Autodesk Inventor part; units mm, degrees
ref_plane "YZ Plane" through (0, 0, 0) normal (1, 0, 0) x (0, 1, 0)
ref_plane "XZ Plane" through (0, 0, 0) normal (0, 1, 0) x (-1, 0, 0)
ref_plane "XY Plane" through (0, 0, 0) normal (0, 0, 1) x (1, 0, 0)
sketch "Náčrt1" plane through (0, 0, 0) normal (0, 0, 1) x (1, 0, 0)
  line L0 (0, 71.1184) -> (0, -73.8108)
  line L1 (-102.6184, 0) -> (105.3108, 0)
  line L2 (-72.5, 50) -> (72.5, 50)
  line L3 (72.5, 50) -> (72.5, -35)
  line L4 (57.5, -50) -> (-72.5, -50)
  line L5 (-72.5, -50) -> (-72.5, 50)
  arc A0 (57.5, -50) -> (72.5, -35) centre (57.5, -35) ccw
  point P0 (0, 0)
  dimension "d2" = 30
  dimension "d37" = 145
  dimension "d38" = 100
extrude "Vysunutí1" add sketch "Náčrt1" along normal blind 21
sketch "Náčrt2" plane through (0, 0, 21) normal (0, 0, 1) x (1, 0, 0)
  line L0 (-72.5, -50) -> (57.5, -50)
  arc A0 (57.5, -50) -> (72.5, -35) centre (57.5, -35) ccw
  line L1 (72.5, -35) -> (72.5, 50)
  line L2 (72.5, 50) -> (-72.5, 50)
  line L3 (-72.5, 50) -> (-72.5, -50)
  circle A1 centre (57.5, -35) radius 15
  line L4 (72.5, -27.3264) -> (72.5, -35)
  line L5 (64.2851, -50) -> (57.5, -50)
  line L6 (72.5, -35) -> (72.5, 50)
  line L7 (72.5, -35) -> (72.5, -35)
  line L8 (72.5, -28.4617) -> (71, -28.4617)
  line L9 (50.9617, -48.5) -> (50.9617, -50)
  point P0 (0, 0)
  point P1 (49.2851, -47.5505)
  point P2 (70.3886, -27.3264)
  point P3 (50.9617, -50)
  dimension "d11" = 1.5
  dimension "d12" = 1.5
extrude "Vysunutí2" cut sketch "Náčrt2" against normal blind 14 contours L9 A1 L0 | A1 A0 | A1 L8 L1
sketch "Náčrt3" plane through (0, 0, 7) normal (0, 0, 1) x (1, 0, 0)
  arc A0 (57.5, -50) -> (72.5, -35) centre (57.5, -35) ccw
  circle A1 centre (57.5, -35) radius 4.25
  line L0 (72.5, -28.4617) -> (72.5, -35)
  line L1 (57.5, -50) -> (50.9617, -50)
  line L2 (71, -28.4617) -> (72.5, -28.4617)
  arc A2 (71, -28.4617) -> (50.9617, -48.5) centre (57.5, -35) ccw
  line L3 (50.9617, -50) -> (50.9617, -48.5)
  point P0 (0, 0)
  dimension "d7" = 8.5
extrude "Vysunutí3" cut sketch "Náčrt3" against normal blind 12 contours A1
fillet "Zaoblení1" radius 2 3 edges at (72.5, 50, 10.5) (-72.5, 50, 10.5) (-72.5, -50, 10.5)
fillet "Zaoblení2" radius 1 2 edges at (71, -28.4617, 14) (50.9617, -48.5, 14)
sketch "Náčrt4" plane through (0, 0, 21) normal (0, 0, 1) x (1, 0, 0)
  arc A0 (50.9617, -49.1129) -> (50.4328, -48.2308) centre (49.9617, -49.1129) ccw
  arc A1 (70.7308, -27.9328) -> (50.4328, -48.2308) centre (57.5, -35) ccw
  arc A2 (70.7308, -27.9328) -> (71.6129, -28.4617) centre (71.6129, -27.4617) ccw
  line L0 (71.6129, -28.4617) -> (72.5, -28.4617)
  line L1 (72.5, -28.4617) -> (72.5, 48)
  arc A3 (72.5, 48) -> (70.5, 50) centre (70.5, 48) ccw
  line L2 (70.5, 50) -> (-70.5, 50)
  arc A4 (-70.5, 50) -> (-72.5, 48) centre (-70.5, 48) ccw
  line L3 (-72.5, 48) -> (-72.5, -48)
  arc A5 (-72.5, -48) -> (-70.5, -50) centre (-70.5, -48) ccw
  line L4 (-70.5, -50) -> (50.9617, -50)
  line L5 (50.9617, -50) -> (50.9617, -49.1129)
  line L6 (-66.5, 44) -> (68.5, 44) construction
  line L7 (68.5, 44) -> (68.5, -44) construction
  line L8 (68.5, -44) -> (-66.5, -44) construction
  line L9 (-66.5, -44) -> (-66.5, 44) construction
  point P0 (0, 0)
  dimension "d14" = 4
  dimension "d15" = 6
  dimension "d16" = 6
  dimension "d17" = 6
sketch "Náčrt5" plane through (0, 0, 21) normal (0, 0, 1) x (1, 0, 0)
  line L0 (-62.1, 26) -> (37.9, 26)
  line L1 (37.9, 26) -> (37.9, -15.5)
  line L2 (37.9, -15.5) -> (-62.1, -15.5)
  line L3 (-62.1, -15.5) -> (-62.1, 26)
  line L4 (-66.5, 44) -> (68.5, 44) construction
  line L5 (-66.5, -44) -> (-66.5, 44) construction
  line L6 (68.5, -44) -> (-66.5, -44) construction
  line L7 (68.5, 44) -> (68.5, -44) construction
  point P0 (0, 0)
  dimension "d18" = 100
  dimension "d19" = 41.5
  dimension "d20" = 18
  dimension "d21" = 4.4
extrude "Vysunutí4" cut sketch "Náčrt5" against normal blind 21
sketch "Náčrt6" plane through (0, 0, 0) normal (0, 0, -1) x (-1, 0, 0)
  line L0 (-37.9, -15.5) -> (-37.9, 26)
  line L1 (-37.9, 26) -> (62.1, 26)
  line L2 (62.1, 26) -> (62.1, -15.5)
  line L3 (62.1, -15.5) -> (-37.9, -15.5)
  arc A0 (70.5, -50) -> (72.5, -48) centre (70.5, -48) ccw
  line L4 (72.5, 48) -> (72.5, -48)
  arc A1 (72.5, 48) -> (70.5, 50) centre (70.5, 48) ccw
  line L5 (-70.5, 50) -> (70.5, 50)
  arc A2 (-70.5, 50) -> (-72.5, 48) centre (-70.5, 48) ccw
  line L6 (-72.5, -35) -> (-72.5, 48)
  arc A3 (-72.5, -35) -> (-57.5, -50) centre (-57.5, -35) ccw
  line L7 (70.5, -50) -> (-57.5, -50)
  circle A4 centre (-57.5, -35) radius 4.25
  arc A5 (-50.4328, -48.2308) -> (-70.7308, -27.9328) centre (-57.5, -35) ccw
  line L8 (0, -73.8108) -> (0, 71.1184)
  line L9 (-105.3108, 0) -> (102.6184, 0)
  line L10 (-68.5, 44) -> (66.5, 44)
  line L11 (66.5, 44) -> (66.5, -44)
  line L12 (66.5, -44) -> (-42.4917, -44)
  line L13 (-68.5, -24.802) -> (-68.5, 44)
  arc A6 (-42.4917, -44) -> (-68.5, -21.3893) centre (-57.5, -35) ccw
  point P0 (0, 0)
  dimension "d24" = 4
  dimension "d25" = 6
  dimension "d26" = 6
  dimension "d27" = 6
  dimension "d28" = 35
extrude "Vysunutí5" cut sketch "Náčrt6" against normal blind 17 contours L3 L8 L12 A6 L13 L9 L0 | L9 L13 L10 L8 L1 L0 | L3 L2 L9 L11 L12 L8 | L8 L10 L11 L9 L2 L1
sketch "Náčrt7" plane through (0, 0, 17) normal (0, 0, -1) x (-1, 0, 0)
  line L0 (-68.5, 44) -> (66.5, 44)
  line L1 (-68.5, -21.3893) -> (-68.5, 44)
  arc A0 (-42.4917, -44) -> (-68.5, -21.3893) centre (-57.5, -35) ccw
  line L2 (66.5, -44) -> (-42.4917, -44)
  line L3 (66.5, 44) -> (66.5, -44)
  line L4 (62.1, -15.5) -> (62.1, 26)
  line L5 (-37.9, -15.5) -> (62.1, -15.5)
  line L6 (-37.9, 26) -> (-37.9, -15.5)
  line L7 (62.1, 26) -> (-37.9, 26)
  line L8 (-40.4, 28.5) -> (64.6, 28.5)
  line L9 (64.6, 28.5) -> (64.6, -18)
  line L10 (64.6, -18) -> (-40.4, -18)
  line L11 (-40.4, -18) -> (-40.4, 28.5)
  point P0 (0, 0)
  dimension "d31" = 2.5
  dimension "d32" = 2.5
  dimension "d33" = 2.5
  dimension "d34" = 2.5
extrude "Vysunutí6" add sketch "Náčrt7" along normal blind 2 contours L8 L9 L10 L11
sketch "Náčrt8" plane through (0, 0, 0) normal (0, 0, -1) x (-1, 0, 0)
  line L0 (-68.5, -21.3893) -> (-68.5, 44)
  line L1 (-68.5, 44) -> (66.5, 44)
  line L2 (66.5, 44) -> (66.5, -44)
  line L3 (66.5, -44) -> (-42.4917, -44)
  arc A0 (-42.4917, -44) -> (-68.5, -21.3893) centre (-57.5, -35) ccw
  arc A1 (70.5, -50) -> (72.5, -48) centre (70.5, -48) ccw
  line L4 (72.5, 48) -> (72.5, -48)
  arc A2 (72.5, 48) -> (70.5, 50) centre (70.5, 48) ccw
  line L5 (-70.5, 50) -> (70.5, 50)
  arc A3 (-70.5, 50) -> (-72.5, 48) centre (-70.5, 48) ccw
  line L6 (-72.5, -35) -> (-72.5, 48)
  arc A4 (-72.5, -35) -> (-57.5, -50) centre (-57.5, -35) ccw
  line L7 (70.5, -50) -> (-57.5, -50)
  circle A5 centre (-57.5, -35) radius 4.25
  point P0 (0, 0)
sketch "Náčrt9" plane through (0, 0, 17) normal (0, 0, -1) x (-1, 0, 0)
  line L0 (-40.4, -18) -> (-40.4, 28.5)
  line L1 (-40.4, 28.5) -> (64.6, 28.5)
  line L2 (64.6, 28.5) -> (64.6, -18)
  line L3 (64.6, -18) -> (-40.4, -18)
  line L4 (-68.5, 44) -> (66.5, 44)
  line L5 (-68.5, -21.3893) -> (-68.5, 44)
  arc A0 (-42.4917, -44) -> (-68.5, -21.3893) centre (-57.5, -35) ccw
  line L6 (66.5, -44) -> (-42.4917, -44)
  line L7 (66.5, 44) -> (66.5, -44)
  line L8 (66.5, -44) -> (-42.4917, -44)
  line L9 (66.5, -44) -> (62, -44)
  line L10 (62, -44) -> (62, -40.5)
  line L11 (62, -40.5) -> (66.5, -40.5)
  line L12 (66.5, -40.5) -> (66.5, -44)
  line L13 (-68.5, 44) -> (-63, 44)
  line L14 (-63, 44) -> (-63, 38.5)
  line L15 (-63, 38.5) -> (-68.5, 38.5)
  line L16 (-68.5, 38.5) -> (-68.5, 44)
  point P0 (0, 0)
  dimension "d48" = 4.5
  dimension "d49" = 3.5
  dimension "d50" = 5.5
  dimension "d51" = 5.5
extrude "Vysunutí7" add sketch "Náčrt9" along normal up to surface (17 mm away) contours L4 L14 L15 L5 | L7 L6 L10 L11
sketch "Náčrt10" plane through (0, 0, 0) normal (0, 0, -1) x (-1, 0, 0)
  circle A0 centre (67, -44.5) radius 3
  circle A1 centre (-68, 45.5) radius 3
  line L0 (-72.5, -35) -> (-72.5, 48)
  line L1 (-70.5, 50) -> (70.5, 50)
  line L2 (70.5, -50) -> (-57.5, -50)
  line L3 (72.5, 48) -> (72.5, -48)
  point P0 (0, 0)
  dimension "d54" = 6
  dimension "d55" = 6
  dimension "d56" = 4.5
  dimension "d57" = 4.5
  dimension "d58" = 5.5
  dimension "d59" = 5.5
sketch "Náčrt11" plane through (0, 0, 21) normal (0, 0, 1) x (1, 0, 0)
  point P0 (0, 0)
  point P1 (-67, -44.5)
  point P2 (68, 45.5)
  point P3 (68, 45.5)
  point P4 (-67, -44.5)
hole "Díra1" at (68, 45.5, 21) at (-67, -44.5, 21) direction (0, 0, -1) diameter 6 depth 17
sketch "Náčrt12" plane through (68, 45.5, 4) normal (0, 0, 1) x (1, 0, 0)
  line L0 (4.5, -73.9617) -> (4.5, 2.5)
  line L1 (2.5, 4.5) -> (-138.5, 4.5)
  circle A0 centre (-135, -90) radius 3
  point P0 (-68, -45.5)
  point P1 (0, 0)
  dimension "d67" = 4.5
  dimension "d68" = 4.5
hole "Díra2" at (68, 45.5, 4) at (-67, -44.5, 4) direction (0, 0, -1) diameter 3.3 depth 17
sketch "Náčrt13" plane through (0, 0, 0) normal (0, 0, -1) x (-1, 0, 0)
  line L0 (49, -47.925) -> (-49, -47.925)
  line L1 (-49, -47.925) -> (-49, -46.075)
  line L2 (-49, -46.075) -> (49, -46.075)
  line L3 (49, -46.075) -> (49, -47.925)
  line L4 (0, -73.8108) -> (0, 71.1184)
  line L5 (70.5, -50) -> (-57.5, -50)
  line L6 (-105.3108, 0) -> (102.6184, 0)
  line L7 (49, 47.925) -> (-49, 47.925)
  line L8 (-49, 47.925) -> (-49, 46.075)
  line L9 (-49, 46.075) -> (49, 46.075)
  line L10 (49, 46.075) -> (49, 47.925)
  line L11 (70.425, -34) -> (68.575, -34)
  line L12 (68.575, -34) -> (68.575, 34)
  line L13 (68.575, 34) -> (70.425, 34)
  line L14 (70.425, 34) -> (70.425, -34)
  line L15 (66.5, 44) -> (66.5, -40.5)
  point P0 (0, 0)
  dimension "d76" = 98
  dimension "d77" = 1.85
  dimension "d78" = 2.075
  dimension "d79" = 1.85
  dimension "d80" = 68
  dimension "d81" = 2.075
extrude "Vysunutí8" add sketch "Náčrt13" along normal blind 9
properties part number "Krabička_horni_3D tisk"
Verification items for the finished model (mm, model axes). A direction names the side the tool comes from. Coordinates: 2 decimals unless noted, no trailing zeros. Order: outer loops, then holes, each group sorted by start corner. A loop starts at its lowest first (then second) coordinate and runs counter-clockwise, first axis right, second up. Notation, with made-up numbers: (31.25, 5.25) - (71.25, 5.25) arc R6 ccw to (71.25, 16.25) - close; hole circle Ø5 at (39.25, -18). An arc over 180 degrees is marked (long way). Return JSON: item names as keys, results as strings.
(1) Section check A-A, the plane x = 23. Record the cut outline in (y, z) (3 decimals).
Filled sheet:
{"outline": "(-50, 0) - (-47.925, 0) - (-47.925, -9) - (-46.075, -9) - (-46.075, 0) - (-44, 0) - (-44, 17) - (-18, 17) - (-18, 15) - (-15.5, 15) - (-15.5, 21) - (-50, 21) - close; (26, 15) - (28.5, 15) - (28.5, 17) - (44, 17) - (44, 0) - (46.075, 0) - (46.075, -9) - (47.925, -9) - (47.925, 0) - (50, 0) - (50, 21) - (26, 21) - close"}
(2) Section check B-B, the plane y = 20. Record the cut outline in (x, z) (3 decimals).
Filled sheet:
{"outline": "(-72.5, 0) - (-70.425, 0) - (-70.425, -9) - (-68.575, -9) - (-68.575, 0) - (-66.5, 0) - (-66.5, 17) - (-64.6, 17) - (-64.6, 15) - (-62.1, 15) - (-62.1, 21) - (-72.5, 21) - close; (37.9, 15) - (40.4, 15) - (40.4, 17) - (68.5, 17) - (68.5, 0) - (72.5, 0) - (72.5, 21) - (37.9, 21) - close"}
(3) Section check D-D, the plane x = 47. Record the cut outline in (y, z) (3 decimals).
Filled sheet:
{"outline": "(-50, 0) - (-47.925, 0) - (-47.925, -9) - (-46.075, -9) - (-46.075, 0) - (-21, 0) - (-21, 17) - (44, 17) - (44, 0) - (46.075, 0) - (46.075, -9) - (47.925, -9) - (47.925, 0) - (50, 0) - (50, 21) - (-24.288, 21) - (-24.288, 7) - (-45.712, 7) - (-45.712, 21) - (-50, 21) - close"}
(4) Go/stop test with flat-tipped pins: pin 1 (4.5 mm diameter, centred on x = 68, y = 45.5, fed in from +Z); pin 2 (3 mm diameter, centred on x = -32, y = 36.5, fed in from -Z); pin 3 (2 mm diameter, centred on x = -69.5, z = -4.5, fed in from +Y). Record where each tip stops, or that it passes through.
Filled sheet:
{"pin 1": "stops at z = 4", "pin 2": "stops at z = 17", "pin 3": "stops at y = 34"}
(5) Thickness scan on line 1 along Y through (x, z) = (57.5, 3); line 2 along X through (y, z) = (24.5, 19.75); line 3 along Y through (x, z) = (25, 18.5). Record the ranges inside material, lowest first.
Filled sheet:
{"line 1": "y = -50 to -39.25, -30.75 to -17.5, 44 to 50", "line 2": "x = -72.5 to -62.1, 37.9 to 72.5", "line 3": "y = -50 to -15.5, 26 to 50"}
(6) Mould release check, pull along X, two halves, no side actions. Record for faces 1 (the flat face through (-70.425, 0, -4)), 2 (the flat face through (-68.575, 0, -4)), 3 (the flat face through (-64, -40.5, 9)): pulls with the +X half, pulls with the -X half, needs draft (parallel to the pull), parting line crosses it, or undercut.
Filled sheet:
{"face 1": "pulls with the -X half", "face 2": "pulls with the +X half", "face 3": "undercut"}
(7) Section check C-C, the plane z = 12.5. Record the cut outline in (x, y).
Filled sheet:
{"outline": "(-72.5, -48) arc R2 ccw to (-70.5, -50) - (50.96, -50) - (50.96, -49.11) arc R1 ccw to (50.43, -48.23) arc R15 cw (long way) to (70.73, -27.93) arc R1 ccw to (71.61, -28.46) - (72.5, -28.46) - (72.5, 48) arc R2 ccw to (70.5, 50) - (-70.5, 50) arc R2 ccw to (-72.5, 48) - close; hole circle Ø6 at (-67, -44.5); hole (-66.5, -40.5) - (-62, -40.5) - (-62, -44) - (42.49, -44) arc R17.5 cw to (68.5, -21.39) - (68.5, 38.5) - (63, 38.5) - (63, 44) - (-66.5, 44) - close; hole circle Ø6 at (68, 45.5)"}
(8) Access from +Z, -Z, +X, -X, +Y, -Y to the whole of each face (thin tool, end or side, straight path). Record for faces 4 (the flat face through (68.5, 8, 8)), 5 (the cylindrical face through (69.8, 47.9, 12.4)), 6 (the flat face through (-1, -47.925, -4)), 7 (the flat face through (1, 46.075, -4)).
Filled sheet:
{"face 4": "-Z", "face 5": "+Z", "face 6": "-Z, +X, -X, -Y", "face 7": "-Z, +X, -X"}
